```python
from build123d import *

# Parameters (mm, degrees)
REVOLVE1_ANGLE     = 45
REVOLVE2_ANGLE     = 2
CUT_EXTRUDE1_DEPTH = 6


with BuildPart() as part:
    # Sketch1 → Revolve1 (revolve, symmetric)
    with BuildSketch(Plane.XY) as revolve1_sk:
        Polygon((97, 0), (97, 5), (124.136396226, 5), (116.717495749, 22.477834241), (127.581099523, 22.477834241), (135, 5), (135, 0), align=None)
    revolve(axis=Axis((0, 0, 0), (0, 1, 0)), revolution_arc=REVOLVE1_ANGLE / 2)
    revolve(revolve1_sk.sketch, axis=Axis((0, 0, 0), (0, -1, 0)), revolution_arc=REVOLVE1_ANGLE / 2)

    # Sketch2 → Revolve2 (revolve)
    with BuildSketch(Plane(origin=(0, 0, 0), x_dir=(0.923879533, 0, 0.382683432), z_dir=(-0.382683432, 0, 0.923879533))):
        Polygon((97, 5), (116.717495749, 22.477834241), (124.136396226, 5), align=None)
    revolve2 = revolve(axis=Axis((0, 0, 0), (0, 1, 0)), revolution_arc=REVOLVE2_ANGLE)

    # Mirror1: Revolve2 across plane
    add(revolve2.mirror(Plane.XY))

    # Sketch3 → Cut-Extrude1 (cut, through all)
    with BuildSketch(Plane(origin=(0, 5, 0), x_dir=(1, 0, 0), z_dir=(0, 1, 0))):
        with BuildLine():
            ThreePointArc((108.183692544, -28.987733051), (112, 0), (108.183692544, 28.987733051))
            ThreePointArc((108.183692544, 28.987733051), (102.059968187, 32.523266957), (98.524434281, 26.3995426))
            ThreePointArc((98.524434281, 26.3995426), (102, 0), (98.524434281, -26.3995426))
            ThreePointArc((98.524434281, -26.3995426), (102.059968187, -32.523266957), (108.183692544, -28.987733051))
        make_face()
    extrude(amount=-CUT_EXTRUDE1_DEPTH, mode=Mode.SUBTRACT)


solid = part.part
```
Here's how the part is built. I have some questions about the finished solid (model axes, mm). A direction names the side the tool comes from. Round coordinates to 2 decimals unless told otherwise and drop trailing zeros. Loops run counter-clockwise (first coordinate to the right, second up) from the corner with the lowest first, then second, coordinate; pieces in that order, holes last. Notation, with made-up numbers: (38.5, -1.75) -> (87.5, -1.75) arc R24 ccw to (87.5, 29.25) -> close; hole circle Ø9 at (28, 72). An arc over 180 degrees is marked (long way). Answer as CSV lines item,"result". Start each with the question number.
1. Imagine slicing it at A-A on y = 19. Write out the boundary of the cut face in (x, z).
2. Imagine slicing it at B-B on x = 100.5. State how many separate pieces and enclosed holes the cut face has, plus the area to 3 significant figures.
3. For faces 5 (the face through (135, 2.5, -0.7)), 6 (the face through (112, 3, 0)), 7 (the face through (97, 2.5, -0.5)), 8 (the face through (99.54, 13.86, -39.24)), 9 (the face through (106.568, 11.919, -39.844)), which set-ups out of +Z, -Z, +X, -X, +Y, -Y let a thin tool reach every point of the face, with its end or its side?
4. I need wall thicknesses on probe 1 along X at (y, z) = (2, -2); probe 2 along Z at (x, y) = (102.5, 12.5); probe 3 along Y at (x, z) = (110.5, 20.5). Which ranges of each line are inside material? Lowest first, please. Write a range as from..to.
5. I'm going to push flat-ended pins straight in: P1, Ø1, axis at x = 103, y = 18, coming from the -Z side; P2, Ø2, axis at y = 13.5, z = 13.5, coming from the -X side; P3, Ø1.5, axis at x = 110, y = 16, coming from the -Z side; P4, Ø3, axis at x = 109, z = -9.5, coming from the +Y side. Where does each tip first touch, or does it pass through?
6. If we mould it in two halves opening along X, with no side actions, what happens to faces 1 (the face through (106.568, 11.919, 39.844)), 2 (the face through (118, 22.478, 1)), 3 (the face through (102, 3, 0)), 4 (the face through (99.54, 13.86, 39.24))? For each: pulls with the +X half, pulls with the -X half, needs draft (parallel to the pull), parting line crosses it, or undercut.
7. Imagine slicing it at C-C on y = 7.25. Write out the boundary of the cut face in (x, z).
Solution:
1,outline,"(104.21, -43.16) -> (119.23, -49.39) arc R129.06 ccw to (119.23, 49.39) -> (104.21, 43.16) arc R112.79 cw to (105.65, 39.5) -> (110.71, 41.39) arc R118.19 cw to (110.71, -41.39) -> (105.65, -39.5) arc R112.79 cw to start"
2,separate pieces,"3"
2,enclosed holes,"0"
2,area,"352 mm²"
3,face 5,"+X, +Y, -Y"
3,face 6,"+Y, -Y"
3,face 7,"-X, +Y, -Y"
3,face 8,"-X, +Y"
3,face 9,"none"
4,probe 1,"96.98..101.98, 111.98..134.99"
4,probe 2,"-42.46..-38.32, 38.32..42.46"
4,probe 3,"0..5"
5,P1,"z = -42.87"
5,P2,"x = 119.33"
5,P3,"z = -45.87"
5,P4,"through"
6,face 1,"undercut"
6,face 2,"needs draft"
6,face 3,"undercut"
6,face 4,"pulls with the -X half"
7,outline,"(91.96, -38.09) -> (123.84, -51.3) arc R134.04 ccw to (123.84, 51.3) -> (91.96, 38.09) arc R99.54 cw to (93.23, 34.86) -> (115.38, 43.14) arc R123.18 cw to (115.38, -43.14) -> (93.23, -34.86) arc R99.54 cw to start"
